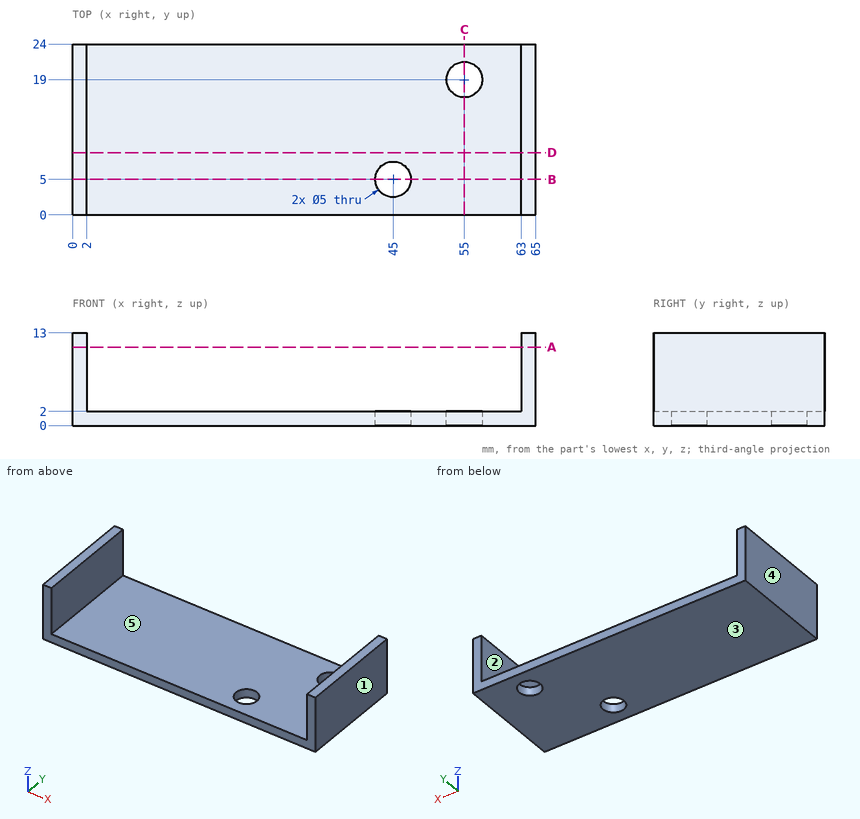
Design review of the part shown in the three views and the two pictorial views. Dimensions are in mm from the part's minimum x, y and z. A direction names the side the tool comes from. Round coordinates to 2 decimals unless told otherwise and drop trailing zeros. Loops run counter-clockwise (first coordinate to the right, second up) from the corner with the lowest first, then second, coordinate; pieces in that order, holes last. Notation, with made-up numbers: (-32, 75.25) -> (16, 75.25) arc R23 ccw to (16, 98.25) -> close; hole circle Ø2 at (20.5, 13). An arc over 180 degrees is marked (long way). Use one line per item in the form item = value. Start each with the question number.
Q1. Machinability: for the marked faces 1 and 2, which of the approach directions +Z, -Z, +X, -X, +Y, -Y give a long, thin tool a straight path to every point of the face, cutting with its end or side? Answer none if there is none.
Q2. We need section C-C on x = 55. Give the boundary of the cut face in (y, z), then the cut area to 3 significant figures.
Q3. We need section D-D on y = 8.75. Give the boundary of the cut face in (x, z), then the cut area to 3 significant figures.
Q4. Draft analysis for pull direction X (two halves, no side actions). For the marked faces 3, 4 and 5, state which applies: +X half, -X half, draft (parallel to the pull), parting line (faces both ways), or undercut.
Q5. For pin 1 Ø3 at (x, y) = (14, 3.5) entering from +Z, flat-tipped, find the tip position at first contact; note if it passes through.
Q6. We need section B-B on y = 5. Give the boundary of the cut face in (x, z), then the cut area to 3 significant figures.
Q7. Wall thickness on line 1 along Y through (x, z) = (45, 1); line 2 along X through (y, z) = (10.5, 3.5); line 3 along Y through (x, z) = (55, 1.5): over which ranges is each line inside the solid? List them lowest first. Write a range as [from, to].
Q8. We need section A-A on z = 11. Give the boundary of the cut face in (x, y), then the cut area to 3 significant figures.
Calculated:
q1.face_1 = +Z, -Z, +X, +Y, -Y
q1.face_2 = +Z, +Y, -Y
q2.outline = (0, 0) -> (16.5, 0) -> (16.5, 2) -> (0, 2) -> close; (21.5, 0) -> (24, 0) -> (24, 2) -> (21.5, 2) -> close
q2.area = 38.0 mm²
q3.outline = (0, 0) -> (65, 0) -> (65, 13) -> (63, 13) -> (63, 2) -> (2, 2) -> (2, 13) -> (0, 13) -> close
q3.area = 174 mm²
q4.face_3 = draft
q4.face_4 = -X half
q4.face_5 = undercut
q5.pin_1 = 2
q6.outline = (0, 0) -> (42.5, 0) -> (42.5, 2) -> (2, 2) -> (2, 13) -> (0, 13) -> close; (47.5, 0) -> (65, 0) -> (65, 13) -> (63, 13) -> (63, 2) -> (47.5, 2) -> close
q6.area = 164 mm²
q7.line_1 = [0, 2.5], [7.5, 24]
q7.line_2 = [0, 2], [63, 65]
q7.line_3 = [0, 16.5], [21.5, 24]
q8.outline = (0, 0) -> (2, 0) -> (2, 24) -> (0, 24) -> close; (63, 0) -> (65, 0) -> (65, 24) -> (63, 24) -> close
q8.area = 96.0 mm²
